from build123d import *

# Parameters (mm, degrees)
SKETCH1_R                                      = 14.2875
BOSS_EXTRUDE1_DEPTH                            = 3.175
SKETCH2_W                                      = 184.202806358
SKETCH2_H                                      = 73.914
CUT_EXTRUDE1_DEPTH                             = 4.175
FILLET1_R                                      = 25.4
SKETCH4_W                                      = 213.36
SKETCH4_H                                      = 64.479988722
CUT_EXTRUDE2_DEPTH                             = 4.175
FILLET2_R                                      = 25.4
SKETCH7_W                                      = 147.610011278
SKETCH7_H                                      = 12.7
CUT_EXTRUDE4_DEPTH                             = 4.175
CSK_FOR_M6_FLAT_HEAD_MACHINE_SCREW1_AT_2_COUNT = 2
CSK_FOR_M6_FLAT_HEAD_MACHINE_SCREW1_AT_2_PITCH = 135.89
CSK_FOR_M6_FLAT_HEAD_MACHINE_SCREW1_AT_3_COUNT = 2
CSK_FOR_M6_FLAT_HEAD_MACHINE_SCREW1_AT_3_PITCH = 229.87
SKETCH10_W                                     = 57.863879914
SKETCH10_H                                     = 74.228534035
CUT_EXTRUDE5_DEPTH                             = 4.175


with BuildPart() as part:
    # Sketch1 → Boss-Extrude1 (new body)
    with BuildSketch(Plane.XY):
        Polygon((-138.259383474, 48.991487021), (32.210627804, -121.478524257), (222.710627804, -121.478524257), (222.710627804, 145.221475743), (-138.259383474, 145.221475743), align=None)
        with Locations((180.538014078, 76.831975743)):
            Circle(SKETCH1_R, mode=Mode.SUBTRACT)
    extrude(amount=BOSS_EXTRUDE1_DEPTH)

    # Sketch2 → Cut-Extrude1 (cut, through all)
    with BuildSketch(Plane.XY.offset(3.175)):
        with Locations((130.662030983, -84.521524257)):
            Rectangle(SKETCH2_W, SKETCH2_H)
    extrude(amount=-CUT_EXTRUDE1_DEPTH, mode=Mode.SUBTRACT)

    # Fillet1
    fillet1_edges = [part.edges().sort_by_distance(p)[0] for p in [
        (38.560627804, -47.564524257, 1.5875),
    ]]
    fillet(fillet1_edges, radius=FILLET1_R)

    # Sketch4 → Cut-Extrude2 (cut, through all)
    with BuildSketch(Plane.XY.offset(3.175)):
        with Locations((-31.579383474, 112.981481382)):
            Rectangle(SKETCH4_W, SKETCH4_H)
    extrude(amount=-CUT_EXTRUDE2_DEPTH, mode=Mode.SUBTRACT)

    # Fillet2
    fillet2_edges = [part.edges().sort_by_distance(p)[0] for p in [
        (-138.259383474, 80.741487021, 1.5875),
        (75.100616526, 80.741487021, 1.5875),
    ]]
    fillet(fillet2_edges, radius=FILLET2_R)

    # Sketch7 → Cut-Extrude4 (cut, through all)
    with BuildSketch(Plane.XY.offset(3.175)):
        with Locations((148.905622165, 138.871475743)):
            Rectangle(SKETCH7_W, SKETCH7_H)
    extrude(amount=-CUT_EXTRUDE4_DEPTH, mode=Mode.SUBTRACT)

    # Sketch8 → CSK for M6 Flat Head Machine Screw1 (revolve, cut)
    with BuildSketch(Plane(origin=(196.040627804, -39.314524257, 0), x_dir=(0, 1, 0), z_dir=(1, 0, 0))):
        Polygon((0, 0), (0, 3.175), (3.3, 3.175), (3.3, 3), (6.3, 0), align=None)
    csk_for_m6_flat_head_machine_screw1 = revolve(axis=Axis((196.040627804, -39.314524257, -6.35), (0, 0, 1)), mode=Mode.SUBTRACT)

    # CSK for M6 Flat Head Machine Screw1 at 2: CSK for M6 Flat Head Machine Screw1 ×2
    with Locations(*[(-i * CSK_FOR_M6_FLAT_HEAD_MACHINE_SCREW1_AT_2_PITCH, 0, 0) for i in range(1, CSK_FOR_M6_FLAT_HEAD_MACHINE_SCREW1_AT_2_COUNT)]):
        add(csk_for_m6_flat_head_machine_screw1, mode=Mode.SUBTRACT)

    # CSK for M6 Flat Head Machine Screw1 at 3: CSK for M6 Flat Head Machine Screw1 ×2
    with Locations(*[(-i * CSK_FOR_M6_FLAT_HEAD_MACHINE_SCREW1_AT_3_PITCH, 0, 0) for i in range(1, CSK_FOR_M6_FLAT_HEAD_MACHINE_SCREW1_AT_3_COUNT)]):
        add(csk_for_m6_flat_head_machine_screw1, mode=Mode.SUBTRACT)

    # Sketch10 → Cut-Extrude5 (cut, through all)
    with BuildSketch(Plane.XY.offset(3.175)):
        with Locations((-131.722312153, 50.636742761)):
            Rectangle(SKETCH10_W, SKETCH10_H)
    extrude(amount=-CUT_EXTRUDE5_DEPTH, mode=Mode.SUBTRACT)


solid = part.part
Part model, mm, in its own coordinate system. Give positions to 0.01 mm unless a question says otherwise; leave off trailing zeros. Order: outer loops, then holes, each group sorted by start corner. A loop starts at its lowest first (then second) coordinate and runs counter-clockwise, first axis right, second up. Notation, with made-up numbers: (60, -26) -> (70, -26) arc R20 cw to (70, -9) -> close; hole circle Ø3 at (-29, 52.25). An arc over 180 degrees is marked (long way). Use one line per item in the form item = value.
(1) Drill centre lines: line 1 (X direction, y = -43, z = 0.45); line 2 (X direction, y = -38, z = 2); line 3 (Y direction, x = 159.5, z = 2.05). Where is each one in solid material? Low to high. Write a range as from..to.
Solution:
line_1 = -46.27..-38.37, -29.29..55.61, 64.69..191.5, 200.58..222.71
line_2 = -51.27..-37.92, -29.74..56.06, 64.24..191.95, 200.13..222.71
line_3 = -47.56..132.52
(2) Pull direction X, two halves, no side cores. Call faces 1 (the face through (170.01, 86.49, 1.57)), 2 (the face through (67.46, 87.98, 1.57)), 3 (the face through (58, 36, 0)): +X half, -X half, draft (parallel to the pull), parting line (faces both ways), or undercut.
Solution:
face_1 = undercut
face_2 = -X half
face_3 = draft
(3) Saw through at A-A (y = 71). Write the cut outline in (x, z) (3 decimals).
Solution:
outline = (-102.79, 0) -> (167.495, 0) -> (167.495, 3.175) -> (-102.79, 3.175) -> close; (193.581, 0) -> (222.711, 0) -> (222.711, 3.175) -> (193.581, 3.175) -> close
(4) Saw through at D-D (x = 93.5). Write the cut outline in (y, z) (3 decimals), then the cut area to 3 significant figures.
Solution:
outline = (-47.565, 0) -> (132.521, 0) -> (132.521, 3.175) -> (-47.565, 3.175) -> close
area = 572 mm²
(5) Saw through at C-C (x = 183.5). Write the cut outline in (y, z) (3 decimals), then the cut area to 3 significant figures.
Solution:
outline = (-47.565, 0) -> (62.855, 0) -> (62.855, 3.175) -> (-47.565, 3.175) -> close; (90.809, 0) -> (132.521, 0) -> (132.521, 3.175) -> (90.809, 3.175) -> close
area = 483 mm²
(6) Flat gauge pin, fed straight in: P1, Ø1.5, axis at x = -11.5, z = 1, coming from the -Y side. Where does the tip first touch, or does it go through?
Solution:
P1 = -78.52
(7) Saw through at B-B (z = 1.85). Count the separate pieces of the cut face and the enclosed holes in it, then the cut area to 3 significant figures.
Solution:
separate_pieces = 1
enclosed_holes = 4
area = 50,200 mm²
